```python
from build123d import *

# Parameters (mm, degrees)
SKETCH2_W                                      = 29
SKETCH2_H                                      = 25
BOSS_EXTRUDE1_DEPTH                            = 6.35
CONVERT_SOLID1_START                           = 3.175
CONVERT_SOLID1_OUTLINE_W                       = 25
CONVERT_SOLID1_OUTLINE_H                       = 29
CONVERT_SOLID1_DEPTH                           = 3.175
CSK_FOR_M3_5_FLAT_HEAD_MACHINE_SCREW1_AT_COUNT = 2
CSK_FOR_M3_5_FLAT_HEAD_MACHINE_SCREW1_AT_PITCH = 12.02081528
CSK_FOR_M3_5_FLAT_HEAD_MACHINE_SCREW_2_COUNT   = 2
CSK_FOR_M3_5_FLAT_HEAD_MACHINE_SCREW_2_PITCH   = 17
CSK_FOR_M3_5_FLAT_HEAD_MACHINE_SCREW_3_COUNT   = 2
CSK_FOR_M3_5_FLAT_HEAD_MACHINE_SCREW_3_PITCH   = 12.02081528
EDGE_FLANGE1_DEPTH                             = 25
EDGE_FLANGE1_BEND_DEPTH                        = 25
SKETCH23_R                                     = 1.95
SKETCH23_R_2                                   = 6.875
BOSS_EXTRUDE2_DEPTH                            = 3.175
FILLET1_R                                      = 40
SKETCH25_R                                     = 1.95
SKETCH25_R_2                                   = 6.875
CUT_EXTRUDE3_DEPTH                             = 107.260166637
FILLET2_R                                      = 2
FILLET3_R                                      = 4
FILLET4_R                                      = 1


with BuildPart() as part:
    # Sketch2 → Boss-Extrude1 (new body)
    with BuildSketch(Plane(origin=(0, 0, 0), x_dir=(0, 0, -1), z_dir=(1, 0, 0))):
        Rectangle(SKETCH2_W, SKETCH2_H)
    extrude(amount=BOSS_EXTRUDE1_DEPTH)

    # Convert-Solid1: read off the stored shape, not the designer's step
    # Convert-Solid1 outline → Convert-Solid1 (cut)
    with BuildSketch(Plane.YZ.offset(CONVERT_SOLID1_START)):
        Rectangle(CONVERT_SOLID1_OUTLINE_W, CONVERT_SOLID1_OUTLINE_H)
    extrude(amount=CONVERT_SOLID1_DEPTH, mode=Mode.SUBTRACT)

    # Sketch4 → CSK for M3.5 Flat Head Machine Screw1 (revolve, cut)
    with BuildSketch(Plane.ZX.offset(-8.5)):
        Polygon((0, 0), (0, 3.175), (1.95, 3.175), (1.95, 2.15), (4.1, 0), align=None)
    csk_for_m3_5_flat_head_machine_screw1 = revolve(axis=Axis((-6.35, -8.5, 0), (1, 0, 0)), mode=Mode.SUBTRACT)

    # CSK for M3.5 Flat Head Machine Screw1 at: CSK for M3.5 Flat Head Machine Screw1 ×2
    with Locations(*[Vector(0, 0.7071067811865476, 0.7071067811865476) * (i * CSK_FOR_M3_5_FLAT_HEAD_MACHINE_SCREW1_AT_PITCH) for i in range(1, CSK_FOR_M3_5_FLAT_HEAD_MACHINE_SCREW1_AT_COUNT)]):
        add(csk_for_m3_5_flat_head_machine_screw1, mode=Mode.SUBTRACT)

    # CSK for M3.5 Flat Head Machine Screw 2: CSK for M3.5 Flat Head Machine Screw1 ×2
    with Locations(*[(0, i * CSK_FOR_M3_5_FLAT_HEAD_MACHINE_SCREW_2_PITCH, 0) for i in range(1, CSK_FOR_M3_5_FLAT_HEAD_MACHINE_SCREW_2_COUNT)]):
        add(csk_for_m3_5_flat_head_machine_screw1, mode=Mode.SUBTRACT)

    # CSK for M3.5 Flat Head Machine Screw 3: CSK for M3.5 Flat Head Machine Screw1 ×2
    with Locations(*[Vector(0, 0.7071067811865476, -0.7071067811865476) * (i * CSK_FOR_M3_5_FLAT_HEAD_MACHINE_SCREW_3_PITCH) for i in range(1, CSK_FOR_M3_5_FLAT_HEAD_MACHINE_SCREW_3_COUNT)]):
        add(csk_for_m3_5_flat_head_machine_screw1, mode=Mode.SUBTRACT)

    # Edge-Flange1: sheet metal written as solids
    # Edge-Flange1 section (on a plane across the edge) → Edge-Flange1 (add)
    with BuildSketch(Plane(origin=(0, 12.5, -17.675), x_dir=(0, 0, 1), z_dir=(0, -1, 0))):
        with BuildLine():
            Line((-3.175, 3.175), (-3.175, 36.825))
            Line((-3.175, 36.825), (0, 36.825))
            Line((0, 36.825), (0, 3.175))
            ThreePointArc((0, 3.175), (0.92993597, 0.92993597), (3.175, 0))
            Line((3.175, 0), (3.175, -3.175))
            ThreePointArc((3.175, -3.175), (-1.315128061, -1.315128061), (-3.175, 3.175))
        make_face()
    extrude(amount=EDGE_FLANGE1_DEPTH)

    # Edge-Flange1 section 2 (on a plane across the edge) → Edge-Flange1 bend (add)
    with BuildSketch(Plane(origin=(0, -12.5, 17.675), x_dir=(0, 0, -1), z_dir=(0, 1, 0))):
        with BuildLine():
            Line((-3.175, 3.175), (-3.175, 36.825))
            Line((-3.175, 36.825), (0, 36.825))
            Line((0, 36.825), (0, 3.175))
            ThreePointArc((0, 3.175), (0.92993597, 0.92993597), (3.175, 0))
            Line((3.175, 0), (3.175, -3.175))
            ThreePointArc((3.175, -3.175), (-1.315128061, -1.315128061), (-3.175, 3.175))
        make_face()
    extrude(amount=EDGE_FLANGE1_BEND_DEPTH)

    # Sketch23 → Boss-Extrude2 (add)
    with BuildSketch(Plane.XY.offset(20.85)):
        with BuildLine():
            Line((-3.175, -12.5), (-3.175, 12.5))
            Line((-3.175, 12.5), (-39.960139618, 76.827855658))
            ThreePointArc((-39.960139618, 76.827855658), (-49.76125368, 80.329282617), (-54.727837027, 71.182978584))
            Line((-54.727837027, 71.182978584), (-36.825, -12.5))
            Line((-36.825, -12.5), (-3.175, -12.5))
        make_face()
        with Locations((-46.90485832, 72.856598659)):
            Circle(SKETCH23_R, mode=Mode.SUBTRACT)
        with Locations((-29.44514168, 27.179817962)):
            Circle(SKETCH23_R, mode=Mode.SUBTRACT)
        with Locations((-38.175, 50.01820831)):
            Circle(SKETCH23_R_2, mode=Mode.SUBTRACT)
    boss_extrude2 = extrude(amount=-BOSS_EXTRUDE2_DEPTH)

    # Mirror3: Boss-Extrude2 across plane
    add(boss_extrude2.mirror(Plane.XY))

    # Fillet1
    fillet1_edges = [part.edges().sort_by_distance(p)[0] for p in [
        (-36.825, -12.5, -19.2625),
        (-36.825, -12.5, 19.2625),
    ]]
    fillet(fillet1_edges, radius=FILLET1_R)

    # Sketch25 → Cut-Extrude3 (cut, through all)
    with BuildSketch(Plane.XY.offset(20.85)):
        with Locations((-46.90485832, 72.856598659)):
            Circle(SKETCH25_R)
        with Locations((-38.175, 50.01820831)):
            Circle(SKETCH25_R_2)
        with Locations((-29.44514168, 27.179817962)):
            Circle(SKETCH25_R)
        with BuildLine():
            Line((-40.030757762, 21.847284007), (-31.33001784, 23.708689176))
            ThreePointArc((-31.33001784, 23.708689176), (-22.681934441, 8.20199276), (-9.994811851, -4.219114299))
            ThreePointArc((-9.994811851, -4.219114299), (-9.344550797, -6.639671437), (-11.568981065, -7.794594065))
            ThreePointArc((-11.568981065, -7.794594065), (-30.444825945, 2.56631328), (-40.030757762, 21.847284007))
        make_face()
        with BuildLine():
            Line((-33.498088379, 29.38063017), (-37.618037608, 40.15892751))
            ThreePointArc((-37.618037608, 40.15892751), (-41.265614485, 40.639310342), (-44.484200888, 42.42152422))
            Line((-44.484200888, 42.42152422), (-41.335566751, 27.703908089))
            Line((-41.335566751, 27.703908089), (-33.498088379, 29.38063017))
        make_face()
        with BuildLine():
            Line((-44.336475361, 57.73519259), (-47.495065423, 65.998455308))
            ThreePointArc((-47.495065423, 65.998455308), (-48.713122103, 66.600238702), (-49.407023256, 65.432203379))
            Line((-49.407023256, 65.432203379), (-47.040106009, 54.368555475))
            ThreePointArc((-47.040106009, 54.368555475), (-45.874551823, 56.201453956), (-44.336475361, 57.73519259))
        make_face()
    extrude(amount=-CUT_EXTRUDE3_DEPTH, mode=Mode.SUBTRACT)

    # Fillet2
    fillet2_edges = [part.edges().sort_by_distance(p)[0] for p in [
        (-40.030757762, 21.847284007, 19.2625),
        (-40.030757762, 21.847284007, -19.2625),
        (-33.498088379, 29.38063017, 19.2625),
        (-41.335566751, 27.703908089, 19.2625),
        (-44.484200888, 42.42152422, 19.2625),
        (-37.618037608, 40.15892751, 19.2625),
        (-33.498088379, 29.38063017, -19.2625),
        (-41.335566751, 27.703908089, -19.2625),
        (-44.484200888, 42.42152422, -19.2625),
        (-37.618037608, 40.15892751, -19.2625),
    ]]
    fillet(fillet2_edges, radius=FILLET2_R)

    # Fillet3
    fillet3_edges = [part.edges().sort_by_distance(p)[0] for p in [
        (-31.33001784, 23.708689176, 19.2625),
        (-31.33001784, 23.708689176, -19.2625),
    ]]
    fillet(fillet3_edges, radius=FILLET3_R)

    # Fillet4
    fillet4_edges = [part.edges().sort_by_distance(p)[0] for p in [
        (-44.336475361, 57.73519259, 19.2625),
        (-47.040106009, 54.368555475, 19.2625),
        (-44.336475361, 57.73519259, -19.2625),
        (-47.040106009, 54.368555475, -19.2625),
    ]]
    fillet(fillet4_edges, radius=FILLET4_R)


solid = part.part
```
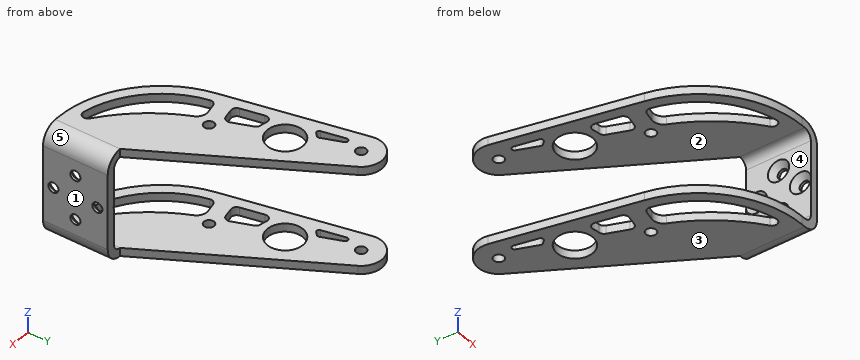
Check sheet for the modelled part. Datum: model origin and axes. Units: mm. Face numbers are marked on the shaded views. A direction names the side the tool comes from. Give positions to 0.01 mm unless a question says otherwise; leave off trailing zeros. Order: outer loops, then holes, each group sorted by start corner. A loop starts at its lowest first (then second) coordinate and runs counter-clockwise, first axis right, second up. Notation, with made-up numbers: M -10.75,61.5 L 0.25,61.5 A10 ccw 0.25,79.5 Z; hole C 57,88 d6. An arc over 180 degrees is marked long. Answer in a Markdown table with one row per item. Add a question column.
Q1. Sectioned sample at B-B, the plane y = 54. Record the boundary of the cut face in (x, z) (3 decimals), and give its area (3 significant figures).
Q2. Sectioned sample at D-D, the plane y = 15. Count the separate pieces of the cut face and the enclosed holes in it, and give its area (3 significant figures).
Q3. Access from +Z, -Z, +X, -X, +Y, -Y to the whole of each face (thin tool, end or side, straight path). Record for the marked faces 4 and 5.
Q4. Sectioned sample at A-A, the plane z = -8.5. Record the boundary of the cut face in (x, y) (3 decimals).
Q5. Sectioned sample at C-C, the plane x = -6.5. Record the boundary of the cut face in (y, z) (3 decimals).
Q6. Gauge pin test, flat ends, axial feed: pin 1 Ø12.5 at (y, z) = (-0.5, 4.5) entering from -X; pin 2 Ø8 at (y, z) = (62.5, -13.5) entering from +X; pin 3 Ø7 at (x, z) = (-1, -3.5) entering from +Y; pin 4 Ø22 at (x, y) = (-38.17, 50.02) entering from -Z. Record the tip position at first contact, or that the pin passes through.
Q7. Thickness scan on L1, parallel to Z at x = -7, y = 14.5 (3 decimals); L2, parallel to Y at x = 2, z = 0; L3, parallel to Y at x = 2.5, z = -8.5. Record the ranges inside material, lowest first.
Q8. Release check for a two-part mould opening along Z. For the marked faces 1, 2 and 3 record: released by +Z, released by -Z, zero draft, split by the parting line, or undercut.
Verdict:
| question | item | result |
|---|---|---|
| 1 | outline | M -51.052,-20.85 L -43.78,-20.85 L -43.78,-17.675 L -51.052,-17.675 Z; M -51.052,17.675 L -43.78,17.675 L -43.78,20.85 L -51.052,20.85 Z; M -32.57,-20.85 L -26.906,-20.85 L -26.906,-17.675 L -32.57,-17.675 Z; M -32.57,17.675 L -26.906,17.675 L -26.906,20.85 L -32.57,20.85 Z |
| 1 | area | 82.1 mm² |
| 2 | separate pieces | 4 |
| 2 | enclosed holes | 0 |
| 2 | area | 170 mm² |
| 3 | face 4 | -X, +Y, -Y |
| 3 | face 5 | +Z, +X, +Y, -Y |
| 4 | outline | M 0,-12.5 L 3.175,-12.5 L 3.175,-1.95 L 2.15,-1.95 L 0,-4.1 Z; M 0,4.1 L 2.15,1.95 L 3.175,1.95 L 3.175,12.5 L 0,12.5 Z |
| 5 | outline | M -12.449,-20.85 L 18.315,-20.85 L 18.315,-17.675 L -12.449,-17.675 Z; M -12.449,17.675 L 18.315,17.675 L 18.315,20.85 L -12.449,20.85 Z |
| 6 | pin 1 | x = 0 |
| 6 | pin 2 | through |
| 6 | pin 3 | y = 12.5 |
| 6 | pin 4 | z = -20.85 |
| 7 | L1 | -20.85 to -17.675, 17.675 to 20.85 |
| 7 | L2 | -12.5 to -10.6, -6.4 to 6.4, 10.6 to 12.5 |
| 7 | L3 | -12.5 to -1.95, 1.95 to 12.5 |
| 8 | face 1 | zero draft |
| 8 | face 2 | undercut |
| 8 | face 3 | released by -Z |
